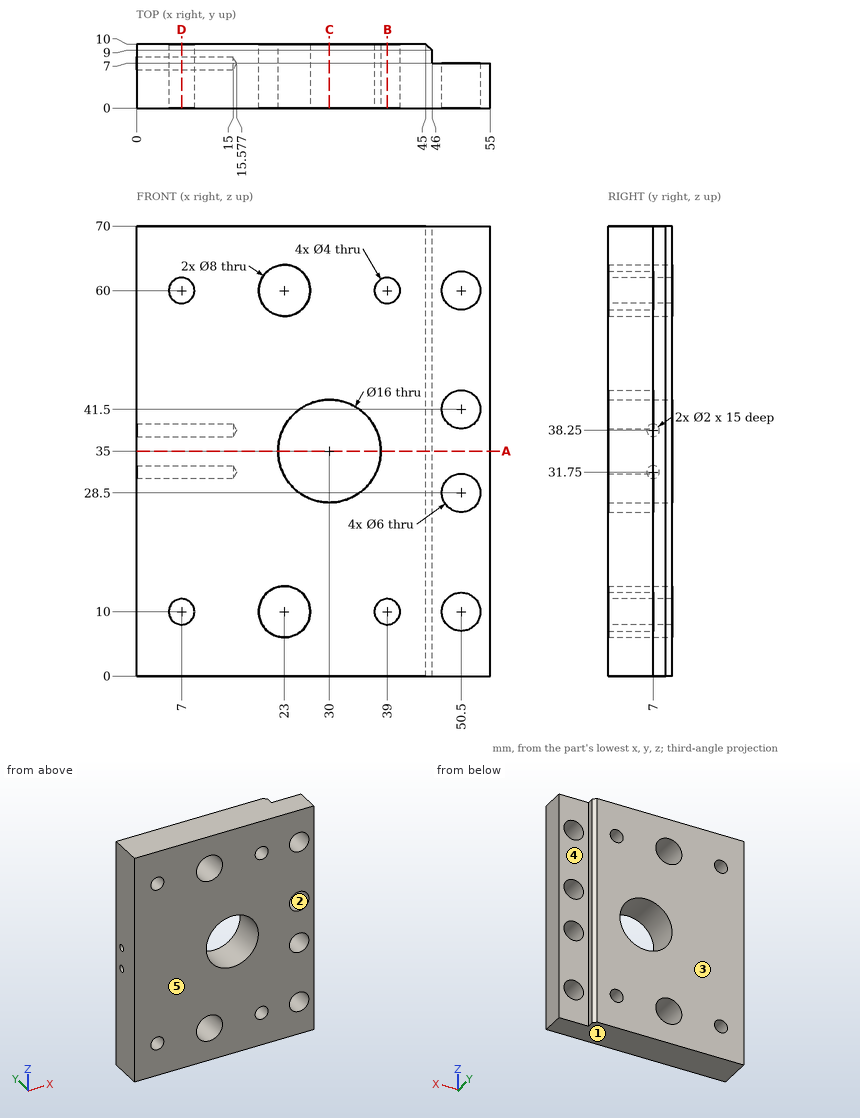
Geometry: see drawing. Coordinates: mm, zero at the bounding-box minimum. A direction names the side the tool comes from. Give positions to 0.01 mm unless a question says otherwise; leave off trailing zeros. Loops run counter-clockwise (first coordinate to the right, second up) from the corner with the lowest first, then second, coordinate; pieces in that order, holes last. Notation, with made-up numbers: (66, 8.25) - (124, 8.25) arc R23 cw to (124, 39.25) - close; hole circle Ø2 at (10, -18.75). An arc over 180 degrees is marked (long way). Use CSV: the item, a comma, the result in double quotes. Start each with the question number.
1. Draft query along Z for the marked faces 1, 2 and 3. Return one class per face: +Z half, -Z half, draft (parallel to the pull), parting line (faces both ways), or undercut.
2. Pin query (flat end, axial travel): pin 1 (1 mm diameter, centred on y = 8, z = 39, fed in from +X). Return the tip coordinate at first contact, or that it passes through.
3. Section D-D (x = 7). Output: boundary loops of the cut face in (y, z), then the cut area to 3 significant figures.
4. Section A-A (z = 35). Output: boundary loops of the cut face in (x, y).
5. Section C-C (x = 30). Output: boundary loops of the cut face in (y, z), then the cut area to 3 significant figures.
6. Ray query, L1, parallel to Z at x = 39, y = 3; L2, parallel to Z at x = 50.5, y = 2.5; L3, parallel to X at y = 2.25, z = 28 (1 decimal). Return the intervals inside material, ascending.
7. Reachability of the marked faces 4 and 5 from +Z, -Z, +X, -X, +Y, -Y: full face, straight path, thin tool, end or side. Return the list, or none.
8. Section B-B (x = 39). Output: boundary loops of the cut face in (y, z).
Response:
1,face 1,"-Z half"
1,face 2,"undercut"
1,face 3,"draft"
2,pin 1,"x = 46"
3,outline,"(0, 0) - (10, 0) - (10, 8) - (0, 8) - close; (0, 12) - (10, 12) - (10, 58) - (0, 58) - close; (0, 62) - (10, 62) - (10, 70) - (0, 70) - close; hole circle Ø2 at (7, 31.75); hole circle Ø2 at (7, 38.25)"
3,area,"614 mm²"
4,outline,"(0, 0) - (22, 0) - (22, 10) - (0, 10) - close; (38, 0) - (55, 0) - (55, 7) - (46, 7) - (46, 9) - (45, 10) - (38, 10) - close"
5,outline,"(0, 0) - (10, 0) - (10, 27) - (0, 27) - close; (0, 43) - (10, 43) - (10, 70) - (0, 70) - close"
5,area,"540 mm²"
6,L1,"0 to 8, 12 to 58, 62 to 70"
6,L2,"0 to 7, 13 to 25.5, 31.5 to 38.5, 44.5 to 57, 63 to 70"
6,L3,"0 to 26.1, 33.9 to 47.5, 53.5 to 55"
7,face 4,"+Z, -Z, +X, +Y"
7,face 5,"+Z, -Z, +X, -X, -Y"
8,outline,"(0, 0) - (10, 0) - (10, 8) - (0, 8) - close; (0, 12) - (10, 12) - (10, 58) - (0, 58) - close; (0, 62) - (10, 62) - (10, 70) - (0, 70) - close"
